from build123d import *

# Parameters (mm, degrees)
F1_W     = 380
F1_H     = 500
F2_DEPTH = 2
F3_W     = 25
F3_H     = 410
F3_W_2   = 410
F3_H_2   = 25
F4_DEPTH = 260


with BuildPart() as f2:
    # F1 (on offset) → F2 (new body)
    with BuildSketch(Plane.XY.offset(258)):
        with Locations((0, -50)):
            Rectangle(F1_W, F1_H)
    extrude(amount=F2_DEPTH)

    # F3 (on Top) → F4 (join)
    with BuildSketch(Plane.XY):
        Rectangle(F3_W, F3_H)
        with Locations((36, 0)):
            Rectangle(F3_W, F3_H)
        with Locations((72, 0)):
            Rectangle(F3_W, F3_H)
        with Locations((108, 0)):
            Rectangle(F3_W, F3_H)
        with Locations((144, 0)):
            Rectangle(F3_W, F3_H)
        with Locations((180, 0)):
            Rectangle(F3_W, F3_H)
        with Locations((-36, 0)):
            Rectangle(F3_W, F3_H)
        with Locations((-72, 0)):
            Rectangle(F3_W, F3_H)
        with Locations((-108, 0)):
            Rectangle(F3_W, F3_H)
        with Locations((-144, 0)):
            Rectangle(F3_W, F3_H)
        with Locations((-180, 0)):
            Rectangle(F3_W, F3_H)
        with Locations((0, -228.5)):
            Rectangle(F3_W_2, F3_H_2)
        with Locations((0, -264.5)):
            Rectangle(F3_W_2, F3_H_2)
        with Locations((0, -300.5)):
            Rectangle(F3_W_2, F3_H_2)
    extrude(amount=F4_DEPTH)


solid = f2.part
Geometry check sheet. Reference: the model listing, model coordinates, mm. A direction names the side the tool comes from. Coordinates: 2 decimals unless noted, no trailing zeros. Order: outer loops, then holes, each group sorted by start corner. A loop starts at its lowest first (then second) coordinate and runs counter-clockwise, first axis right, second up. Notation, with made-up numbers: (79, 17.5) - (120, 17.5) arc R8 cw to (120, 26.5) - close; hole circle Ø7 at (82, 13). An arc over 180 degrees is marked (long way). Answer in a Markdown table with one row per item. Add a question column.
1) Release check for a two-part mould opening along X. For faces 4 (the flat face through (-95.5, -3, 128)), 5 (the flat face through (205, -265, 128)), 6 (the flat face through (-144, -205, 127)), 7 (the flat face through (59.5, -3, 128)) record: +X half, -X half, draft (parallel to the pull), parting line (faces both ways), or undercut.
2) Gauge pin test, flat ends, axial feed: P1, Ø0.6, axis at y = -248, z = 259, coming from the +X side; P2, Ø10, axis at y = 107, z = 102.5, coming from the -X side; P3, Ø1, axis at y = -208.5, z = 259, coming from the -X side. Record the tip position at first contact, or that the pin passes through.
3) Set-up check for faces 1 (the flat face through (144, -205, 127)), 2 (the flat face through (-12.5, -3, 128)), 3 (the flat face through (192.5, -3, 128)): record each of +Z, -Z, +X, -X, +Y, -Y from which the full face is reachable in a straight line by a thin tool's end or side.
4) Material ranges on line 1 along Y through (x, z) = (-76.5, 200); line 2 along Y through (x, z) = (158, 228); line 3 along Z through (x, y) = (-157.5, 115.5), recorded low to high. Write a range as [from, to].
5) Cross-section at B-B, the plane z = 55. State how many separate pieces and enclosed holes the cut face has, then the cut area to 4 significant figures.
6) Cross-section at A-A, the plane x = 109. Record the cut outline in (y, z), then the cut area to 3 significant figures.
Check result:
| question | item | result |
|---|---|---|
| 1 | face 4 | undercut |
| 1 | face 5 | +X half |
| 1 | face 6 | draft |
| 1 | face 7 | undercut |
| 2 | P1 | stops at x = 190 |
| 2 | P2 | stops at x = -192.5 |
| 2 | P3 | stops at x = -190 |
| 3 | face 1 | -Z, +X, -X |
| 3 | face 2 | -Z, +Y |
| 3 | face 3 | +Z, -Z, +X, +Y |
| 4 | line 1 | y = [-313, -288], [-277, -252], [-241, -216], [-205, 205] |
| 4 | line 2 | y = [-313, -288], [-277, -252], [-241, -216] |
| 4 | line 3 | z = [258, 260] |
| 5 | separate pieces | 14 |
| 5 | enclosed holes | 0 |
| 5 | area | 143,500 mm² |
| 6 | outline | (-313, 0) - (-288, 0) - (-288, 258) - (-277, 258) - (-277, 0) - (-252, 0) - (-252, 258) - (-241, 258) - (-241, 0) - (-216, 0) - (-216, 258) - (-205, 258) - (-205, 0) - (205, 0) - (205, 260) - (-313, 260) - close |
| 6 | area | 126,000 mm² |
